```python
from build123d import *

# Parameters (mm, degrees)
SKETCH_1_W          = 102
SKETCH_1_H          = 67
EXTRUDE_1_DEPTH     = 2
SKETCH_2_R          = 1.6
CUT_EXTRUDE_1_DEPTH = 123.05326706
FILLET_1_R          = 1
SKETCH_3_R          = 1.65
SKETCH_3_W          = 10
SKETCH_3_H          = 3.95
SKETCH_3_W_2        = 11
SKETCH_3_H_2        = 11
CUT_EXTRUDE_2_DEPTH = 123.05326706
FILLET_2_R          = 1
FILLET_3_R          = 0.6
FILLET_4_R          = 0.5


with BuildPart() as part:
    # 草图1 → 凸台-拉伸1 (new body)
    with BuildSketch(Plane.XY):
        with Locations((51, 33.5)):
            Rectangle(SKETCH_1_W, SKETCH_1_H)
    extrude(amount=EXTRUDE_1_DEPTH)

    # 草图2 → 切除-拉伸1 (cut, through all)
    with BuildSketch(Plane.XY.offset(2)):
        with Locations((3.5, 63.5)):
            Circle(SKETCH_2_R)
        with Locations((98.5, 63.5)):
            Circle(SKETCH_2_R)
        with Locations((98.5, 3.5)):
            Circle(SKETCH_2_R)
        with Locations((3.5, 3.5)):
            Circle(SKETCH_2_R)
    extrude(amount=-CUT_EXTRUDE_1_DEPTH, mode=Mode.SUBTRACT)

    # 圆角1
    fillet_1_edges = [part.edges().sort_by_distance(p)[0] for p in [
        (0, 67, 1),
        (102, 67, 1),
        (102, 0, 1),
        (0, 0, 1),
    ]]
    fillet(fillet_1_edges, radius=FILLET_1_R)

    # 草图3 → 切除-拉伸2 (cut, through all)
    with BuildSketch(Plane.XY.offset(2)):
        with Locations((35, 60)):
            Circle(SKETCH_3_R)
        with Locations((67, 60)):
            Circle(SKETCH_3_R)
        with Locations((67, 28)):
            Circle(SKETCH_3_R)
        with Locations((35, 28)):
            Circle(SKETCH_3_R)
        with Locations((80.8, 11.175)):
            Rectangle(SKETCH_3_W, SKETCH_3_H)
        with Locations((45.9, 11.175)):
            Rectangle(SKETCH_3_W, SKETCH_3_H)
        with Locations((21.3, 14.7)):
            Rectangle(SKETCH_3_W_2, SKETCH_3_H_2)
        with BuildLine():
            Line((52.5, 42.5), (70.191469459, 42.5))
            ThreePointArc((70.191469459, 42.5), (64.611805538, 30.388194462), (52.5, 24.808530541))
            Line((52.5, 24.808530541), (52.5, 42.5))
        make_face()
        with BuildLine():
            Line((31.808530541, 45.5), (49.5, 45.5))
            Line((49.5, 45.5), (49.5, 63.191469459))
            ThreePointArc((49.5, 63.191469459), (37.388194462, 57.611805538), (31.808530541, 45.5))
        make_face()
        with BuildLine():
            Line((31.808530541, 42.5), (49.5, 42.5))
            Line((49.5, 42.5), (49.5, 24.808530541))
            ThreePointArc((49.5, 24.808530541), (37.388194462, 30.388194462), (31.808530541, 42.5))
        make_face()
        with BuildLine():
            Line((52.5, 63.191469459), (52.5, 45.5))
            Line((52.5, 45.5), (70.191469459, 45.5))
            ThreePointArc((70.191469459, 45.5), (64.611805538, 57.611805538), (52.5, 63.191469459))
        make_face()
    extrude(amount=-CUT_EXTRUDE_2_DEPTH, mode=Mode.SUBTRACT)

    # 圆角2
    fillet_2_edges = [part.edges().sort_by_distance(p)[0] for p in [
        (70.191469459, 42.5, 1),
        (52.5, 24.808530541, 1),
        (52.5, 42.5, 1),
        (31.808530541, 45.5, 1),
        (49.5, 63.191469459, 1),
        (49.5, 45.5, 1),
        (31.808530541, 42.5, 1),
        (49.5, 42.5, 1),
        (52.5, 63.191469459, 1),
        (70.191469459, 45.5, 1),
        (52.5, 45.5, 1),
    ]]
    fillet(fillet_2_edges, radius=FILLET_2_R)

    # 圆角3
    fillet_3_edges = [part.edges().sort_by_distance(p)[0] for p in [
        (75.8, 9.2, 1),
        (75.8, 13.15, 1),
        (85.8, 13.15, 1),
        (85.8, 9.2, 1),
        (40.9, 9.2, 1),
        (40.9, 13.15, 1),
        (50.9, 13.15, 1),
        (50.9, 9.2, 1),
    ]]
    fillet(fillet_3_edges, radius=FILLET_3_R)

    # 圆角4
    fillet_4_edges = [part.edges().sort_by_distance(p)[0] for p in [
        (26.8, 20.2, 1),
        (26.8, 9.2, 1),
        (15.8, 9.2, 1),
        (15.8, 20.2, 1),
    ]]
    fillet(fillet_4_edges, radius=FILLET_4_R)


solid = part.part
```
The model under review builds one solid part; all positions refer to its coordinate system, in mm. A direction names the side the tool comes from. Round coordinates to 2 decimals unless told otherwise and drop trailing zeros. Order: outer loops, then holes, each group sorted by start corner. A loop starts at its lowest first (then second) coordinate and runs counter-clockwise, first axis right, second up.
Item 1: Draft analysis for pull direction X (two halves, no side actions). For faces 1 (the flat face through (0, 33, 1)), 2 (the flat face through (52.5, 54, 1)), 3 (the flat face through (50, 34, 2)), state which applies: released by +X, released by -X, zero draft, split by the parting line, or undercut.
Working result:
face 1: released by -X
face 2: undercut
face 3: zero draft
Item 2: Add section D-D, the plane x = 35. State the section outline as (y, z) points.
Working result:
outline: (0, 0) - (26.35, 0) - (26.35, 2) - (0, 2) - close; (29.65, 0) - (33.3, 0) - (33.3, 2) - (29.65, 2) - close; (42.5, 0) - (45.5, 0) - (45.5, 2) - (42.5, 2) - close; (54.7, 0) - (58.35, 0) - (58.35, 2) - (54.7, 2) - close; (61.65, 0) - (67, 0) - (67, 2) - (61.65, 2) - close
Item 3: Machinability: for faces 4 (the flat face through (50, 67, 1)), 5 (the flat face through (75.8, 11, 1)), which of the approach directions +Z, -Z, +X, -X, +Y, -Y give a long, thin tool a straight path to every point of the face, cutting with its end or side? Answer none if there is none.
Working result:
face 4: +Z, -Z, +X, -X, +Y
face 5: +Z, -Z
Item 4: Add section A-A, the plane x = 3.5. State the section outline as (y, z) points, and give its area (3 significant figures).
Working result:
outline: (0, 0) - (1.9, 0) - (1.9, 2) - (0, 2) - close; (5.1, 0) - (61.9, 0) - (61.9, 2) - (5.1, 2) - close; (65.1, 0) - (67, 0) - (67, 2) - (65.1, 2) - close
area: 121 mm2
Item 5: Add section C-C, the plane y = 28. State the section outline as (x, z) points.
Working result:
outline: (0, 0) - (33.35, 0) - (33.35, 2) - (0, 2) - close; (36.65, 0) - (40.3, 0) - (40.3, 2) - (36.65, 2) - close; (49.5, 0) - (52.5, 0) - (52.5, 2) - (49.5, 2) - close; (61.7, 0) - (65.35, 0) - (65.35, 2) - (61.7, 2) - close; (68.65, 0) - (102, 0) - (102, 2) - (68.65, 2) - close
Item 6: Add section B-B, the plane y = 3.5. State the section outline as (x, z) points.
Working result:
outline: (0, 0) - (1.9, 0) - (1.9, 2) - (0, 2) - close; (5.1, 0) - (96.9, 0) - (96.9, 2) - (5.1, 2) - close; (100.1, 0) - (102, 0) - (102, 2) - (100.1, 2) - close
Item 7: For pin 1 (3 mm diameter, centred on x = 98.5, y = 3.5, fed in from -Z), flat-tipped, find the tip position at first contact; note if it passes through.
Working result:
pin 1: passes through
Item 8: To check wall thickness, follow probe 1 along Y at (x, z) = (3.5, 1.55); probe 2 along Y at (x, z) = (62, 1.3); probe 3 along Y at (x, z) = (20, 1.75). State the ranges of each line that lie inside material, in increasing order.
Working result:
probe 1: y = 0 to 1.9, 5.1 to 61.9, 65.1 to 67
probe 2: y = 0 to 28.2, 42.5 to 45.5, 59.8 to 67
probe 3: y = 0 to 9.2, 20.2 to 67
